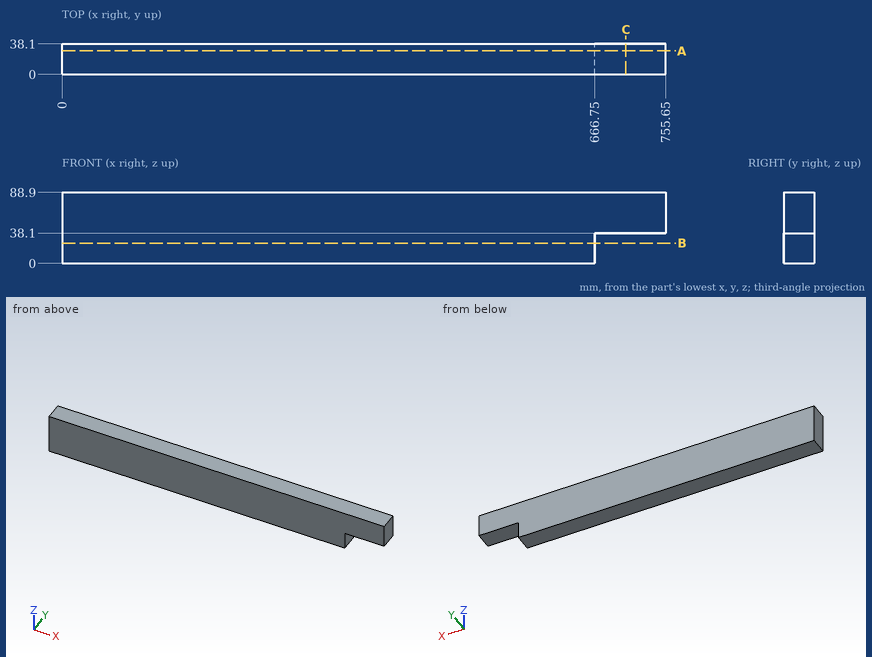
Job drawing, mm, ordinate dimensions from the low corner. One solid piece. Give positions to 0.01 mm unless a question says otherwise; leave off trailing zeros. Order: outer loops, then holes, each group sorted by start corner. A loop starts at its lowest first (then second) coordinate and runs counter-clockwise, first axis right, second up. Notation, with made-up numbers: (83.5, 12) - (105.5, 12) arc R15 ccw to (105.5, 19) - close; hole circle Ø5 at (77, 9). An arc over 180 degrees is marked (long way). Return JSON: item names as keys, results as strings.
1) Cut at A-A, the plane y = 29.5. Give the cut face in (x, z), plus the area to 3 significant figures.
Geometry says:
{"outline": "(0, 0) - (666.75, 0) - (666.75, 38.1) - (755.65, 38.1) - (755.65, 88.9) - (0, 88.9) - close", "area": "63,800 mm²"}
2) Cut at B-B, the plane z = 25.5. Give the cut face in (x, y), plus the area to 3 significant figures.
Geometry says:
{"outline": "(0, 0) - (666.75, 0) - (666.75, 38.1) - (0, 38.1) - close", "area": "25,400 mm²"}
3) Flat gauge pin, fed straight in: P1, Ø19, axis at y = 10, z = 28, coming from the +X side. Where does the tip first touch, or does it go through?
Geometry says:
{"P1": "x = 666.75"}
4) Probe line 1 (X direction, y = 35.5, z = 20.5); line 2 (Z direction, x = 677.5, y = 23.5). List the from-to ranges inside material, lowest first. Write a range as from..to.
Geometry says:
{"line 1": "0..666.75", "line 2": "38.1..88.9"}
5) Cut at C-C, the plane x = 706. Give the cut face in (y, z), plus the area to 3 significant figures.
Geometry says:
{"outline": "(0, 38.1) - (38.1, 38.1) - (38.1, 88.9) - (0, 88.9) - close", "area": "1,940 mm²"}
